```python
from build123d import *

# Parameters (mm, degrees)
SKETCH1_R           = 38.5
SKETCH1_R_2         = 14
BOSS_EXTRUDE1_DEPTH = 8
SKETCH2_W           = 16
SKETCH2_H           = 62.340339885
BOSS_EXTRUDE2_DEPTH = 8
FILLET1_R           = 4
SKETCH3_W           = 12.5
SKETCH3_H           = 2
SKETCH4_W           = 1.3
SKETCH4_H           = 0.7
SKETCH5_R           = 23
SKETCH5_R_2         = 21
BOSS_EXTRUDE3_DEPTH = 2
SKETCH6_R           = 2.15
CUT_EXTRUDE1_DEPTH  = 109.343204678
CIRPATTERN1_COUNT   = 8
SKETCH7_R           = 3
CUT_EXTRUDE2_DEPTH  = 111.735044137


with BuildPart() as part:
    # Sketch1 → Boss-Extrude1 (new, symmetric)
    with BuildSketch(Plane.XY):
        Circle(SKETCH1_R)
        Circle(SKETCH1_R_2, mode=Mode.SUBTRACT)
    extrude(amount=BOSS_EXTRUDE1_DEPTH, both=True)

    # Sketch2 → Boss-Extrude2 (add, symmetric)
    with BuildSketch(Plane.XY):
        with Locations((0, 68.829830058)):
            Rectangle(SKETCH2_W, SKETCH2_H)
    extrude(amount=BOSS_EXTRUDE2_DEPTH, both=True)

    # Fillet1
    fillet1_edges = [part.edges().sort_by_distance(p)[0] for p in [
        (-8, 37.659660115, 0),
        (8, 37.659660115, 0),
    ]]
    fillet(fillet1_edges, radius=FILLET1_R)

    # Sketch3 → Cut-Revolve1 (revolve, cut)
    with BuildSketch(Plane(origin=(0, 0, 0), x_dir=(0, 0, -1), z_dir=(1, 0, 0)), mode=Mode.PRIVATE) as cut_revolve1_sk:
        with Locations((-1.75, 15)):
            Rectangle(SKETCH3_W, SKETCH3_H)
    revolve(cut_revolve1_sk.sketch.rotate(Axis((0, 0, 0), (0, 0, -1)), 90), axis=Axis((0, 0, 0), (0, 0, -1)), mode=Mode.SUBTRACT)

    # Sketch4 → Cut-Revolve2 (revolve, cut)
    with BuildSketch(Plane(origin=(0, 0, 0), x_dir=(0, 0, -1), z_dir=(1, 0, 0)), mode=Mode.PRIVATE) as cut_revolve2_sk:
        with Locations((-5.05, 16.35)):
            Rectangle(SKETCH4_W, SKETCH4_H)
    revolve(cut_revolve2_sk.sketch.rotate(Axis((0, 0, 0), (0, 0, -1)), 90), axis=Axis((0, 0, 0), (0, 0, -1)), mode=Mode.SUBTRACT)

    # Sketch5 → Boss-Extrude3 (add)
    with BuildSketch(Plane(origin=(0, 0, -8), x_dir=(-1, 0, 0), z_dir=(0, 0, -1))):
        with Locations(Location((0, 0, 0), (0, 0, 180))):
            Circle(SKETCH5_R)
        Circle(SKETCH5_R_2, mode=Mode.SUBTRACT)
    extrude(amount=BOSS_EXTRUDE3_DEPTH)

    # Sketch6 → Cut-Extrude1 (cut, through all)
    with BuildSketch(Plane(origin=(0, 0, -8), x_dir=(-1, 0, 0), z_dir=(0, 0, -1))):
        with Locations((0, 33.5)):
            Circle(SKETCH6_R)
    cut_extrude1 = extrude(amount=-CUT_EXTRUDE1_DEPTH, mode=Mode.SUBTRACT)

    # CirPattern1: Cut-Extrude1 ×8 about axis, 2 skipped
    cirpattern1_axis = Axis((0, 0, 0), (0, 0, 1))
    add([cut_extrude1.rotate(cirpattern1_axis, i * 360 / CIRPATTERN1_COUNT) for i in range(1, CIRPATTERN1_COUNT) if i not in (2, 6)], mode=Mode.SUBTRACT)

    # Sketch7 → Cut-Extrude2 (cut, through all)
    with BuildSketch(Plane(origin=(8, 0, 0), x_dir=(0, 0, -1), z_dir=(1, 0, 0))):
        with Locations(Location((0, 90, 0), (0, 0, 90))):
            Circle(SKETCH7_R)
        with Locations(Location((0, 70, 0), (0, 0, 90))):
            Circle(SKETCH7_R)
    extrude(amount=-CUT_EXTRUDE2_DEPTH, mode=Mode.SUBTRACT)


solid = part.part
```
Design review of the part built by this model. Coordinates are the model's own, in mm. A direction names the side the tool comes from. Coordinates: 2 decimals unless noted, no trailing zeros. Loops run counter-clockwise (first coordinate to the right, second up) from the corner with the lowest first, then second, coordinate; pieces in that order, holes last. Notation, with made-up numbers: (38, 0) - (54, 0) arc R31 ccw to (54, 29) - close; hole circle Ø5 at (84, -21). An arc over 180 degrees is marked (long way). Use CSV: the item, a comma, the result in double quotes. Start each with the question number.
1) Wall thickness on L1, parallel to Y at x = 0, z = -6.6; L2, parallel to X at y = 0.5, z = -6.75; L3, parallel to Z at x = 2.5, y = 70: over which ranges is each line inside the solid? List them lowest first. Write a range as from..to.
2) Consider section D-D on y = -18. Write out the cut boundary in (x, z), then the cut area to 3 significant figures.
3) Tool access review of faces 4 (the cylindrical face through (8.78, 38.4, 0.11)), 5 (the flat face through (4, -14, -8)), 6 (the flat face through (0.07, 14.15, -4.5)), 7 (the cylindrical face through (-2.17, -16.56, 5.04)): name each direction out of +Z, -Z, +X, -X, +Y, -Y from which nothing blocks a thin tool from reaching the whole face with its end or side.
4) For pin 1 Ø1 at (x, z) = (-19, 2.5) entering from -Y; pin 2 Ø5 at (x, y) = (-12.5, 39) entering from -Z; pin 3 Ø8 at (y, z) = (78, -2) entering from -X, all flat-tipped, find the tip position at first contact; note any pin that passes through.
5) Consider section A-A on y = 90. Write out the cut boundary in (x, z), then the cut area to 3 significant figures.
6) Consider section B-B on z = 0. Give the number of separate pieces and of enclosed holes in the cut face, then the cut area to 3 significant figures.
7) The part is to be moulded in two halves that separate along X. For faces 1 (the cylindrical face through (-3.47, 15.62, -0.11)), 2 (the flat face through (-8, 70, 4)), 3 (the cylindrical face through (0, 87, 0)), say which applies: +X half, -X half, draft (parallel to the pull), parting line (faces both ways), or undercut.
Geometry says:
1,L1,"-38.5..-35.65, -31.35..-14, 14..31.35, 35.65..100"
1,L2,"-38.5..-13.99, 13.99..38.5"
1,L3,"-8..-3, 3..8"
2,outline,"(-34.03, -8) - (-14.32, -8) - (-14.32, -10) - (-10.82, -10) - (-10.82, -8) - (10.82, -8) - (10.82, -10) - (14.32, -10) - (14.32, -8) - (34.03, -8) - (34.03, 8) - (-34.03, 8) - close"
2,area,"1,100 mm^2"
3,face 4,"+Z, -Z, +X, +Y"
3,face 5,"-Z"
3,face 6,"+Z"
3,face 7,"none"
4,pin 1,"y = -33.76"
4,pin 2,"z = -8"
4,pin 3,"x = -8"
5,outline,"(-8, -8) - (8, -8) - (8, -3) - (-8, -3) - close; (-8, 3) - (8, 3) - (8, 8) - (-8, 8) - close"
5,area,"160 mm^2"
6,separate pieces,"3"
6,enclosed holes,"7"
6,area,"4,570 mm^2"
7,face 1,"undercut"
7,face 2,"-X half"
7,face 3,"draft"
